```python
from build123d import *

# Parameters (mm, degrees)
SKETCH1_R           = 9.525
SKETCH1_R_2         = 3.175
BOSS_EXTRUDE1_DEPTH = 8.382
SKETCH2_R           = 6.35
SKETCH2_R_2         = 3.175
BOSS_EXTRUDE2_DEPTH = 6.604
SKETCH3_R           = 9.525
SKETCH3_R_2         = 3.175
BOSS_EXTRUDE3_DEPTH = 8.382


with BuildPart() as part:
    # Sketch1 → Boss-Extrude1 (new body)
    with BuildSketch(Plane(origin=(0, 0, 0), x_dir=(0, 0, -1), z_dir=(1, 0, 0))):
        Circle(SKETCH1_R)
        Circle(SKETCH1_R_2, mode=Mode.SUBTRACT)
    extrude(amount=BOSS_EXTRUDE1_DEPTH)

    # Sketch2 → Boss-Extrude2 (add)
    with BuildSketch(Plane(origin=(8.382, 0, 0), x_dir=(0, 0, -1), z_dir=(1, 0, 0))):
        with Locations(Location((0, 0, 0), (0, 0, 180))):
            Circle(SKETCH2_R)
        Circle(SKETCH2_R_2, mode=Mode.SUBTRACT)
    extrude(amount=BOSS_EXTRUDE2_DEPTH)

    # Sketch3 → Boss-Extrude3 (add)
    with BuildSketch(Plane(origin=(14.986, 0, 0), x_dir=(0, 0, -1), z_dir=(1, 0, 0))):
        Circle(SKETCH3_R)
        Circle(SKETCH3_R_2, mode=Mode.SUBTRACT)
    extrude(amount=BOSS_EXTRUDE3_DEPTH)


solid = part.part
```
Build history of the part. All positions in model axes, mm. A direction names the side the tool comes from. Give positions to 0.01 mm unless a question says otherwise; leave off trailing zeros. Loops run counter-clockwise (first coordinate to the right, second up) from the corner with the lowest first, then second, coordinate; pieces in that order, holes last. Notation, with made-up numbers: (-25, 78.25) - (-13, 78.25) arc R17 cw to (-13, 111.25) - close; hole circle Ø3 at (73, -32). An arc over 180 degrees is marked (long way). Use a Markdown table: item, result.
(1) Band-saw the part on B-B (z = -1). Give the cut face in (x, y).
Taken from the geometry:
| item | result |
|---|---|
| outline | (0, -9.47) - (8.38, -9.47) - (8.38, -6.27) - (14.99, -6.27) - (14.99, -9.47) - (23.37, -9.47) - (23.37, -3.01) - (0, -3.01) - close; (0, 3.01) - (23.37, 3.01) - (23.37, 9.47) - (14.99, 9.47) - (14.99, 6.27) - (8.38, 6.27) - (8.38, 9.47) - (0, 9.47) - close |
(2) Pull direction X, two halves, no side cores. Call faces 3 (the face through (23.368, 0, -4)), 4 (the face through (11.52, -3.1, 0.69)), 5 (the face through (8.382, -6.2, -2)): +X half, -X half, draft (parallel to the pull), parting line (faces both ways), or undercut.
Taken from the geometry:
| item | result |
|---|---|
| face 3 | +X half |
| face 4 | draft |
| face 5 | undercut |
(3) Band-saw the part on D-D (y = -6.75). Give the cut face in (x, z).
Taken from the geometry:
| item | result |
|---|---|
| outline | (0, -6.72) - (8.38, -6.72) - (8.38, 6.72) - (0, 6.72) - close; (14.99, -6.72) - (23.37, -6.72) - (23.37, 6.72) - (14.99, 6.72) - close |
(4) Which spindle directions (+Z, -Z, +X, -X, +Y, -Y) get a long thin tool onto all of the face, cutting with end or side? Do faces 1 (the face through (4.132, -5.796, 7.559)), 2 (the face through (11.638, 5.634, 2.93)). Say none if no direction does.
Taken from the geometry:
| item | result |
|---|---|
| face 1 | +X, -X |
| face 2 | none |
(5) Band-saw the part on A-A (y = 0). Give the cut face in (x, z) (3 decimals).
Taken from the geometry:
| item | result |
|---|---|
| outline | (0, -9.525) - (8.382, -9.525) - (8.382, -6.35) - (14.986, -6.35) - (14.986, -9.525) - (23.368, -9.525) - (23.368, -3.175) - (0, -3.175) - close; (0, 3.175) - (23.368, 3.175) - (23.368, 9.525) - (14.986, 9.525) - (14.986, 6.35) - (8.382, 6.35) - (8.382, 9.525) - (0, 9.525) - close |
(6) Band-saw the part on C-C (x = 11). Give the cut face in (y, z) (3 decimals), and give its area (3 significant figures).
Taken from the geometry:
| item | result |
|---|---|
| outline | circle Ø12.7 at (0, 0); hole circle Ø6.35 at (0, 0) |
| area | 95.0 mm2 |
(7) Drop flat-ended pins along their axis: pin 1 Ø10 at (x, z) = (12.5, -7) entering from +Y; pin 2 Ø2 at (x, y) = (6, -6.5) entering from -Z; pin 3 Ø6 at (x, y) = (15.5, 4.5) entering from -Z. Give the stop position or say it passes through.
Taken from the geometry:
| item | result |
|---|---|
| pin 1 | y = 9.15 |
| pin 2 | z = -7.78 |
| pin 3 | z = -9.41 |
(8) Wall check: line 1 along Y through (x, z) = (10, 0) (3 decimals); line 2 along X through (y, z) = (-7, 6); line 3 along Y through (x, z) = (17.25, 0) (3 decimals). Give the ranges that are in metal, low to high.
Taken from the geometry:
| item | result |
|---|---|
| line 1 | -6.35 to -3.175, 3.175 to 6.35 |
| line 2 | 0 to 8.38, 14.99 to 23.37 |
| line 3 | -9.525 to -3.175, 3.175 to 9.525 |
